from build123d import *

# Parameters (mm, degrees)
PAD_START       = 56
PAD_DEPTH       = 38
SKETCH001_R     = 18.7
POCKET_DEPTH    = 34
SKETCH002_R     = 6.2
SKETCH002_R_2   = 1.6
POCKET001_DEPTH = 4
POCKET002_DEPTH = 45.401
SKETCH004_R     = 3.2
POCKET003_DEPTH = 3.6
SKETCH005_R     = 6
POCKET004_DEPTH = 1


with BuildPart() as part:
    # Sketch → Pad (new body)
    with BuildSketch(Plane.XZ.offset(PAD_START)):
        with BuildLine():
            Line((37.3, 1), (37.3, -53))
            ThreePointArc((37.3, -53), (60, -75.7), (82.7, -53))
            Line((82.7, -53), (82.7, 1))
            ThreePointArc((82.7, 1), (81.82132, 3.12132), (79.7, 4))
            Line((79.7, 4), (40.3, 4))
            ThreePointArc((40.3, 4), (38.17868, 3.12132), (37.3, 1))
        make_face()
    extrude(amount=PAD_DEPTH)

    # Sketch001 (on Face7 of Pad) → Pocket (cut)
    with BuildSketch(Plane(origin=(0, -56, 0), x_dir=(1, 0, 0), z_dir=(0, 1, 0))):
        with Locations((60, 53)):
            Circle(SKETCH001_R)
    extrude(amount=-POCKET_DEPTH, mode=Mode.SUBTRACT)

    # Sketch002 (on Face5 of Pocket) → Pocket001 (cut)
    with BuildSketch(Plane.XZ.offset(94)):
        with Locations((60, -60)):
            Circle(SKETCH002_R)
        with Locations((52.25, -39.576606)):
            Circle(SKETCH002_R_2)
        with Locations((67.75, -39.576606)):
            Circle(SKETCH002_R_2)
        with Locations((75.5, -53)):
            Circle(SKETCH002_R_2)
        with Locations((67.75, -66.423394)):
            Circle(SKETCH002_R_2)
        with Locations((52.25, -66.423394)):
            Circle(SKETCH002_R_2)
        with Locations((44.5, -53)):
            Circle(SKETCH002_R_2)
    extrude(amount=-POCKET001_DEPTH, mode=Mode.SUBTRACT)

    # Sketch003 (on Face7 of Pocket001) → Pocket002 (cut, through all)
    with BuildSketch(Plane(origin=(82.7, 0, 0), x_dir=(0, 0, 1), z_dir=(1, 0, 0))):
        with BuildLine():
            Line((-30.4, 87.4), (-30.4, 62.6))
            ThreePointArc((-30.4, 62.6), (-29.52132, 60.47868), (-27.4, 59.6))
            Line((-27.4, 59.6), (-2.6, 59.6))
            ThreePointArc((-2.6, 59.6), (-0.47868, 60.47868), (0.4, 62.6))
            Line((0.4, 62.6), (0.4, 87.4))
            ThreePointArc((0.4, 87.4), (-0.47868, 89.52132), (-2.6, 90.4))
            Line((-2.6, 90.4), (-27.4, 90.4))
            ThreePointArc((-27.4, 90.4), (-29.52132, 89.52132), (-30.4, 87.4))
        make_face()
    extrude(amount=-POCKET002_DEPTH, mode=Mode.SUBTRACT)

    # Sketch004 (on Face14 of Pocket002) → Pocket003 (cut)
    with BuildSketch(Plane(origin=(0, 0, 4), x_dir=(-1, 0, 0), z_dir=(0, 0, 1))):
        with Locations((-70, 75)):
            Circle(SKETCH004_R)
        with Locations((-50, 75)):
            Circle(SKETCH004_R)
    extrude(amount=-POCKET003_DEPTH, mode=Mode.SUBTRACT)

    # Sketch005 (on Face14 of Pocket003) → Pocket004 (cut)
    with BuildSketch(Plane(origin=(0, 0, 4), x_dir=(-1, 0, 0), z_dir=(0, 0, 1))):
        with Locations((-70, 75)):
            Circle(SKETCH005_R)
        with Locations((-50, 75)):
            Circle(SKETCH005_R)
    extrude(amount=-POCKET004_DEPTH, mode=Mode.SUBTRACT)


solid = part.part
Geometry check sheet. Reference: the model listing, model coordinates, mm. A direction names the side the tool comes from. Round coordinates to 2 decimals unless told otherwise and drop trailing zeros. Order: outer loops, then holes, each group sorted by start corner. A loop starts at its lowest first (then second) coordinate and runs counter-clockwise, first axis right, second up. Notation, with made-up numbers: M 74.5,5.25 L 122.5,5.25 A27 ccw 122.5,23.25 Z; hole C 3,19.5 d2. An arc over 180 degrees is marked long. Answer in a Markdown table with one row per item.
(1) Sectioned sample at D-D, the plane y = -74. Record the cut outline in (x, z), and give its area (3 significant figures).
Responses:
| item | result |
|---|---|
| outline | M 37.3,-53 A22.7 ccw 82.7,-53 L 82.7,-30.4 L 37.3,-30.4 Z; M 37.3,0.4 L 46.96,0.4 L 46.96,3 L 44.08,3 L 44.08,4 L 40.3,4 A3 ccw 37.3,1 Z; M 53.04,0.4 L 66.96,0.4 L 66.96,3 L 64.08,3 L 64.08,4 L 55.92,4 L 55.92,3 L 53.04,3 Z; M 73.04,0.4 L 82.7,0.4 L 82.7,1 A3 ccw 79.7,4 L 75.92,4 L 75.92,3 L 73.04,3 Z; hole C 60,-53 d37.4 |
| area | 841 mm² |
(2) Draft check along Z on faces 1 (the face through (37.3, -75, -38)), 2 (the face through (77.026, -92.028, -52.519)), 3 (the face through (67, -72, 3)). Enter one of: released by +Z, released by -Z, zero draft, split by the parting line, or undercut.
Responses:
| item | result |
|---|---|
| face 1 | zero draft |
| face 2 | undercut |
| face 3 | released by +Z |
(3) Go/stop test with flat-tipped pins: P1, Ø9.5, axis at x = 50, y = -75, coming from the +Z side; P2, Ø12, axis at x = 65, y = -68.5, coming from the -Z side; P3, Ø12.5, axis at x = 70.5, y = -70.5, coming from the -Z side; P4, Ø1, axis at y = -68.5, z = -29, coming from the -X side. Record where each tip stops, or that it passes through.
Responses:
| item | result |
|---|---|
| P1 | stops at z = 3 |
| P2 | stops at z = -75.7 |
| P3 | stops at z = -75.3 |
| P4 | passes through |
(4) Scan lines: probe 1 along Z at (x, y) = (60, -64); probe 2 along X at (y, z) = (-75, 1); probe 3 along Y at (x, z) = (43, -2.5). Record each from-to range of solid material in increasing order. Write a range as from..to.
Responses:
| item | result |
|---|---|
| probe 1 | z = -75.7..-71.7, -34.3..-30.4, 0.4..4 |
| probe 2 | x = 37.3..46.8, 53.2..66.8, 73.2..82.7 |
| probe 3 | y = -94..-90.4, -59.6..-56 |
(5) Sectioned sample at C-C, the plane z = -26. Record the cut outline in (x, y).
Responses:
| item | result |
|---|---|
| outline | M 37.3,-94 L 82.7,-94 L 82.7,-90.4 L 37.3,-90.4 Z; M 37.3,-59.6 L 82.7,-59.6 L 82.7,-56 L 37.3,-56 Z |
(6) Sectioned sample at B-B, the plane y = -66.5. Record the cut outline in (x, z), and give its area (3 significant figures).
Responses:
| item | result |
|---|---|
| outline | M 37.3,-53 A22.7 ccw 82.7,-53 L 82.7,-30.4 L 37.3,-30.4 Z; M 37.3,0.4 L 82.7,0.4 L 82.7,1 A3 ccw 79.7,4 L 40.3,4 A3 ccw 37.3,1 Z; hole C 60,-53 d37.4 |
| area | 896 mm² |
(7) Sectioned sample at A-A, the plane x = 60. Record the cut outline in (y, z).
Responses:
| item | result |
|---|---|
| outline | M -94,-75.7 L -56,-75.7 L -56,-71.7 L -90,-71.7 L -90,-66.2 L -94,-66.2 Z; M -94,-53.8 L -90,-53.8 L -90,-34.3 L -56,-34.3 L -56,4 L -94,4 Z; hole M -90.4,-27.4 A3 ccw -87.4,-30.4 L -62.6,-30.4 A3 ccw -59.6,-27.4 L -59.6,-2.6 A3 ccw -62.6,0.4 L -87.4,0.4 A3 ccw -90.4,-2.6 Z |
(8) Tool access check on faces 4 (the face through (50.694, -71.876, 1.718)), 5 (the face through (60, -75, 0.4)), 6 (the face through (60, -90, -53)). Record the directions out of +Z, -Z, +X, -X, +Y, -Y that give a thin tool (end or side, any length) a straight path to the whole face; none if there is none.
Responses:
| item | result |
|---|---|
| face 4 | +Z |
| face 5 | +X, -X |
| face 6 | +Y |
